```python
from build123d import *

# Parameters (mm, degrees)
SKETCH002_AS_DRAWN_W                 = 76
SKETCH002_AS_DRAWN_H                 = 50
SKETCH002_AS_DRAWN_R                 = 3.5
EXTRUDE003_DEPTH                     = 3.5
EXTRUDE003_ONTO_SKETCH002_ROLL_ANGLE = 90
CYLINDER_R                           = 16.25
CYLINDER_DEPTH                       = 10
SKETCH_R                             = 14
EXTRUDE001_DEPTH                     = 13
CYLINDER001_R                        = 16.25
CYLINDER001_DEPTH                    = 10
EXTRUDE_DEPTH                        = 13
SKETCH001_AS_DRAWN_W                 = 40
SKETCH001_AS_DRAWN_H                 = 70
EXTRUDE002_DEPTH                     = 21
EXTRUDE002_ONTO_SKETCH001_ROLL_ANGLE = 90


with BuildPart() as extrude003:
    # Sketch002 as drawn → Extrude003 (new)
    with BuildSketch(Plane.XY):
        Rectangle(SKETCH002_AS_DRAWN_W, SKETCH002_AS_DRAWN_H)
        with Locations((-32.5, 0)):
            Circle(SKETCH002_AS_DRAWN_R, mode=Mode.SUBTRACT)
        with Locations((32.5, 0)):
            Circle(SKETCH002_AS_DRAWN_R, mode=Mode.SUBTRACT)
    extrude(amount=-EXTRUDE003_DEPTH)


with BuildPart() as extrude003_1:
    # Extrude003 onto Sketch002 roll: moved
    add(extrude003.part.rotate(Axis((0, 0, 0), (1, 0, 0)), EXTRUDE003_ONTO_SKETCH002_ROLL_ANGLE))


with BuildPart() as extrude003_2:
    # Extrude003 onto Sketch002 placement: moved
    add(extrude003_1.part)


with BuildPart() as extrude003_3:
    # Extrude003 placement: moved
    add(extrude003_2.part.moved(Location((0, -45, 0))))


with BuildPart() as cylinder:
    # Cylinder → Cylinder (new body)
    with BuildSketch(Plane.XY):
        Circle(CYLINDER_R)
    extrude(amount=CYLINDER_DEPTH)


with BuildPart() as obj1:
    # Sketch → Extrude001 (new body)
    with BuildSketch(Plane.XY):
        with BuildLine():
            ThreePointArc((20, 0), (0, 20), (-20, 0))
            Line((-20, 0), (-20, -35))
            Line((-20, -35), (20, -35))
            Line((20, -35), (20, 0))
        make_face()
        Circle(SKETCH_R, mode=Mode.SUBTRACT)
    extrude(amount=EXTRUDE001_DEPTH)

    # Cut: cut Cylinder
    add(cylinder.part, mode=Mode.SUBTRACT)


with BuildPart() as obj1_1:
    # Cut placement: moved
    add(obj1.part.moved(Location((0, 0, -35))))


with BuildPart() as cylinder001:
    # Cylinder001 → Cylinder001 (new body)
    with BuildSketch(Plane.XY.offset(3)):
        Circle(CYLINDER001_R)
    extrude(amount=CYLINDER001_DEPTH)


with BuildPart() as bearing_nest_r_cut:
    # Sketch → Extrude (new body)
    with BuildSketch(Plane.XY):
        with BuildLine():
            ThreePointArc((20, 0), (0, 20), (-20, 0))
            Line((-20, 0), (-20, -35))
            Line((-20, -35), (20, -35))
            Line((20, -35), (20, 0))
        make_face()
        Circle(SKETCH_R, mode=Mode.SUBTRACT)
    extrude(amount=EXTRUDE_DEPTH)

    # Cut001: cut Cylinder001
    add(cylinder001.part, mode=Mode.SUBTRACT)


with BuildPart() as bearing_nest_r_cut_1:
    # Cut001 placement: moved
    add(bearing_nest_r_cut.part.moved(Location((0, 0, 22))))


with BuildPart() as fusion:
    # Sketch001 as drawn → Extrude002 (new)
    with BuildSketch(Plane.XY):
        Rectangle(SKETCH001_AS_DRAWN_W, SKETCH001_AS_DRAWN_H)
    extrude(amount=-EXTRUDE002_DEPTH)


with BuildPart() as fusion_1:
    # Extrude002 onto Sketch001 roll: moved
    add(fusion.part.rotate(Axis((0, 0, 0), (1, 0, 0)), EXTRUDE002_ONTO_SKETCH001_ROLL_ANGLE))


with BuildPart() as fusion_2:
    # Extrude002 onto Sketch001 placement: moved
    add(fusion_1.part)


with BuildPart() as fusion_3:
    # Extrude002 placement: moved
    add(fusion_2.part.moved(Location((0, -45, 0))))

    # Fusion: union Extrude003, obj1, bearing-nest-r-cut
    add(extrude003_3.part)
    add(obj1_1.part)
    add(bearing_nest_r_cut_1.part)


solid = fusion_3.part
```
CAD build for the part. Positions are in the model's coordinates, mm. A direction names the side the tool comes from. Coordinates: 2 decimals unless noted, no trailing zeros. Order: outer loops, then holes, each group sorted by start corner. A loop starts at its lowest first (then second) coordinate and runs counter-clockwise, first axis right, second up. Notation, with made-up numbers: (33.5, -36) -> (42.5, -36) arc R24 ccw to (42.5, -23) -> close; hole circle Ø7 at (51.5, 5.5). An arc over 180 degrees is marked (long way). Use one line per item in the form item = value. Start each with the question number.
1) Drop flat-ended pins along their axis: pin 1 (12 mm diameter, centred on x = 0.5, z = -9, fed in from +Y); pin 2 (3 mm diameter, centred on x = -33, y = -43.5, fed in from -Z); pin 3 (4 mm diameter, centred on x = -30.5, y = -42.5, fed in from +Z); pin 4 (6.5 mm diameter, centred on x = 32.5, z = 0, fed in from -Y). Give the stop position or say it passes through.
2) Pull direction Z, two halves, no side cores. Call faces 1 (the flat face through (29, -43, 25)), 2 (the cylindrical face through (0, 20, -29)), 3 (the flat face through (-13.3, 4.9, -25)), 4 (the flat face through (0, -24, 0)): +Z half, -Z half, draft (parallel to the pull), parting line (faces both ways), or undercut.
3) Band-saw the part on B-B on x = 0. Give the cut face in (y, z), then the cut area to 3 significant figures.
4) Tool access for faces 5 (the cylindrical face through (15.5, 4.88, 29.93)), 6 (the cylindrical face through (15.5, 4.88, -30.07)), 7 (the flat face through (27, -41.5, 0)): list every direction of +Z, -Z, +X, -X, +Y, -Y with a clear straight run to the whole face (end or side of a thin tool).
5) Band-saw the part on A-A on z = -23.5. Give the cut face in (x, y), then the cut area to 3 significant figures.
6) Band-saw the part on D-D on x = -32.5. Give the cut face in (y, z), then the cut area to 4 significant figures.
7) Drill centre lines: L1, parallel to Z at x = 6, y = -19; L2, parallel to Y at x = 0, z = 30; L3, parallel to Z at x = 32.5, y = -43.5. Where is each one in solid material? Low to high. Write a range as [from, to].
8) Band-saw the part on C-C on y = -5.5. Give the cut face in (x, z).
Entries:
q1.pin_1 = -24
q1.pin_2 = -25
q1.pin_3 = 25
q1.pin_4 = through
q2.face_1 = +Z half
q2.face_2 = draft
q2.face_3 = -Z half
q2.face_4 = undercut
q3.outline = (-45, -35) -> (-16.25, -35) -> (-16.25, -25) -> (-14, -25) -> (-14, -22) -> (-24, -22) -> (-24, 22) -> (-14, 22) -> (-14, 25) -> (-16.25, 25) -> (-16.25, 35) -> (-45, 35) -> close; (14, -25) -> (16.25, -25) -> (16.25, -35) -> (20, -35) -> (20, -22) -> (14, -22) -> close; (14, 22) -> (20, 22) -> (20, 35) -> (16.25, 35) -> (16.25, 25) -> (14, 25) -> close
q3.area = 1,800 mm2
q4.face_5 = +Z
q4.face_6 = -Z
q4.face_7 = +Z, -Z, +X, +Y
q5.outline = (-38, -45) -> (38, -45) -> (38, -41.5) -> (20, -41.5) -> (20, 0) arc R20 ccw to (-20, 0) -> (-20, -41.5) -> (-38, -41.5) -> close; hole circle Ø28 at (0, 0)
q5.area = 1,940 mm2
q6.outline = (-45, -25) -> (-41.5, -25) -> (-41.5, -3.5) -> (-45, -3.5) -> close; (-45, 3.5) -> (-41.5, 3.5) -> (-41.5, 25) -> (-45, 25) -> close
q6.area = 150.5 mm2
q7.L1 = [-35, -22], [22, 35]
q7.L2 = [-45, -16.25], [16.25, 20]
q7.L3 = [-25, -3.5], [3.5, 25]
q8.outline = (-20, -35) -> (-15.29, -35) -> (-15.29, -25) -> (-12.87, -25) -> (-12.87, -22) -> (-20, -22) -> close; (-20, 22) -> (-12.87, 22) -> (-12.87, 25) -> (-15.29, 25) -> (-15.29, 35) -> (-20, 35) -> close; (12.87, -25) -> (15.29, -25) -> (15.29, -35) -> (20, -35) -> (20, -22) -> (12.87, -22) -> close; (12.87, 22) -> (20, 22) -> (20, 35) -> (15.29, 35) -> (15.29, 25) -> (12.87, 25) -> close
